```python
from build123d import *

# Parameters (mm, degrees)
SKETCH1_W           = 50
SKETCH1_H           = 21
BOSS_EXTRUDE1_DEPTH = 58
SKETCH3_R           = 7.5
CUT_EXTRUDE1_DEPTH  = 24
CUT_EXTRUDE2_REACH  = 66.025
SKETCH4_R           = 5.2
CUT_EXTRUDE3_START  = -24
SKETCH5_R           = 7.5
CUT_EXTRUDE3_DEPTH  = 24
CUT_EXTRUDE4_REACH  = 66.025
SKETCH6_R           = 4.5
CUT_EXTRUDE5_REACH  = 68.558
SKETCH8_W           = 10
SKETCH8_H           = 20
SKETCH11_W          = 4
SKETCH11_H          = 20
BOSS_EXTRUDE2_DEPTH = 26
SKETCH12_W          = 18
SKETCH12_H          = 20
BOSS_EXTRUDE3_DEPTH = 4
CUT_EXTRUDE7_DEPTH  = 79.487260113
FILLET1_R           = 5
SKETCH14_R          = 1.95
CUT_EXTRUDE8_DEPTH  = 10
SKETCH15_W          = 5.527864045
SKETCH15_H          = 1
CUT_EXTRUDE9_DEPTH  = 76.028327984
SKETCH17_W          = 30
SKETCH17_H          = 19
BOSS_EXTRUDE5_DEPTH = 18
SKETCH7_R           = 4.125
CUT_EXTRUDE6_DEPTH  = 45
FILLET8_R           = 3
SKETCH18_W          = 6
SKETCH18_H          = 5.5
CUT_EXTRUDE10_DEPTH = 1


with BuildPart() as part:
    # Sketch1 → Boss-Extrude1 (new body)
    with BuildSketch(Plane(origin=(0, 0, 0), x_dir=(1, 0, 0), z_dir=(0, 1, 0))):
        Rectangle(SKETCH1_W, SKETCH1_H)
    extrude(amount=BOSS_EXTRUDE1_DEPTH)

    # Sketch3 → Cut-Extrude1 (cut)
    with BuildSketch(Plane(origin=(0, 58, 0), x_dir=(1, 0, 0), z_dir=(0, 1, 0))):
        with Locations(Location((-15, 0, 0), (0, 0, 270))):
            Circle(SKETCH3_R)
    extrude(amount=-CUT_EXTRUDE1_DEPTH, mode=Mode.SUBTRACT)

    # Sketch4 → Cut-Extrude2 (cut, up to next)
    with BuildSketch(Plane(origin=(0, 58, 0), x_dir=(1, 0, 0), z_dir=(0, 1, 0)), mode=Mode.PRIVATE) as cut_extrude2_sk1:
        with Locations(Location((15, 0, 0), (0, 0, 270))):
            Circle(SKETCH4_R)
    cut_extrude2_tool1 = extrude(cut_extrude2_sk1.sketch, amount=-CUT_EXTRUDE2_REACH, mode=Mode.PRIVATE) & part.part
    add(cut_extrude2_tool1.solids().sort_by_distance((15, 58, 0))[0], mode=Mode.SUBTRACT)

    # Sketch5 → Cut-Extrude3 (cut)
    with BuildSketch(Plane.XZ.offset(CUT_EXTRUDE3_START)):
        with Locations(Location((-15, 0, 0), (0, 0, 90))):
            Circle(SKETCH5_R)
    extrude(amount=CUT_EXTRUDE3_DEPTH, mode=Mode.SUBTRACT)

    # Sketch6 → Cut-Extrude4 (cut, up to next)
    with BuildSketch(Plane.XZ, mode=Mode.PRIVATE) as cut_extrude4_sk1:
        with Locations(Location((-15, 0, 0), (0, 0, 270))):
            Circle(SKETCH6_R)
    cut_extrude4_tool1 = extrude(cut_extrude4_sk1.sketch, amount=-CUT_EXTRUDE4_REACH, mode=Mode.PRIVATE) & part.part
    add(cut_extrude4_tool1.solids().sort_by_distance((-15, 0, 0))[0], mode=Mode.SUBTRACT)

    # Sketch8 → Cut-Extrude5 (cut, up to next)
    with BuildSketch(Plane.XY.offset(10.5), mode=Mode.PRIVATE) as cut_extrude5_sk1:
        with Locations((0, 29)):
            Rectangle(SKETCH8_W, SKETCH8_H)
    cut_extrude5_tool1 = extrude(cut_extrude5_sk1.sketch, amount=-CUT_EXTRUDE5_REACH, mode=Mode.PRIVATE) & part.part
    add(cut_extrude5_tool1.solids().sort_by_distance((0, 29, 10.5))[0], mode=Mode.SUBTRACT)

    # Sketch11 → Boss-Extrude2 (add)
    with BuildSketch(Plane(origin=(0, 0, -10.5), x_dir=(-1, 0, 0), z_dir=(0, 0, -1))):
        with Locations((7, 29)):
            Rectangle(SKETCH11_W, SKETCH11_H)
        with Locations((-7, 29)):
            Rectangle(SKETCH11_W, SKETCH11_H)
    extrude(amount=BOSS_EXTRUDE2_DEPTH)

    # Sketch12 → Boss-Extrude3 (add)
    with BuildSketch(Plane(origin=(0, 0, -36.5), x_dir=(-1, 0, 0), z_dir=(0, 0, -1))):
        with Locations((0, 29)):
            Rectangle(SKETCH12_W, SKETCH12_H)
    extrude(amount=BOSS_EXTRUDE3_DEPTH)

    # Sketch13 → Cut-Extrude7 (cut, through all)
    with BuildSketch(Plane(origin=(9, 0, 0), x_dir=(0, 0, -1), z_dir=(1, 0, 0))):
        with BuildLine():
            Line((18.25, 31.75), (27.25, 31.75))
            ThreePointArc((27.25, 31.75), (30, 29), (27.25, 26.25))
            Line((27.25, 26.25), (18.25, 26.25))
            ThreePointArc((18.25, 26.25), (15.5, 29), (18.25, 31.75))
        make_face()
    extrude(amount=-CUT_EXTRUDE7_DEPTH, mode=Mode.SUBTRACT)

    # Fillet1
    fillet1_edges = [part.edges().sort_by_distance(p)[0] for p in [
        (25, 29, 10.5),
        (-25, 29, 10.5),
    ]]
    fillet(fillet1_edges, radius=FILLET1_R)

    # Sketch14 → Cut-Extrude8 (cut)
    with BuildSketch(Plane.XZ):
        with Locations(Location((20.550788232, 5.550788232, 0), (0, 0, 270))):
            Circle(SKETCH14_R)
        with Locations(Location((9.449211768, -5.550788232, 0), (0, 0, 270))):
            Circle(SKETCH14_R)
    extrude(amount=-CUT_EXTRUDE8_DEPTH, mode=Mode.SUBTRACT)

    # Sketch15 → Cut-Extrude9 (cut, through all)
    with BuildSketch(Plane(origin=(0, 58, 0), x_dir=(1, 0, 0), z_dir=(0, 1, 0))):
        with Locations((-22.236067977, 0)):
            Rectangle(SKETCH15_W, SKETCH15_H)
    extrude(amount=-CUT_EXTRUDE9_DEPTH, mode=Mode.SUBTRACT)

    # Sketch17 → Boss-Extrude5 (add)
    with BuildSketch(Plane(origin=(9, 0, 0), x_dir=(0, 0, -1), z_dir=(1, 0, 0))):
        with Locations((25.5, 48.5)):
            Rectangle(SKETCH17_W, SKETCH17_H)
        with Locations((25.5, 9.5)):
            Rectangle(SKETCH17_W, SKETCH17_H)
    extrude(amount=-BOSS_EXTRUDE5_DEPTH)

    # Sketch7 → Cut-Extrude6 (cut)
    with BuildSketch(Plane.XY.offset(10.5)):
        with Locations((0, 49)):
            Circle(SKETCH7_R)
        with Locations((0, 9)):
            Circle(SKETCH7_R)
    extrude(amount=-CUT_EXTRUDE6_DEPTH, mode=Mode.SUBTRACT)

    # Fillet8
    fillet8_edges = [part.edges().sort_by_distance(p)[0] for p in [
        (-9, 29, -40.5),
        (9, 29, -40.5),
    ]]
    fillet(fillet8_edges, radius=FILLET8_R)

    # Sketch18 → Cut-Extrude10 (cut)
    with BuildSketch(Plane(origin=(0, 0, -40.5), x_dir=(-1, 0, 0), z_dir=(0, 0, -1))):
        with Locations((0, 29)):
            Rectangle(SKETCH18_W, SKETCH18_H)
    extrude(amount=-CUT_EXTRUDE10_DEPTH, mode=Mode.SUBTRACT)


solid = part.part
```
The model under review builds one solid part; all positions refer to its coordinate system, in mm. A direction names the side the tool comes from. Round coordinates to 2 decimals unless told otherwise and drop trailing zeros. Order: outer loops, then holes, each group sorted by start corner. A loop starts at its lowest first (then second) coordinate and runs counter-clockwise, first axis right, second up. Notation, with made-up numbers: (-11.5, 38.25) - (43.5, 38.25) arc R22 ccw to (43.5, 76.25) - close; hole circle Ø5 at (-3, -32). An arc over 180 degrees is marked (long way). Answer in a Markdown table with one row per item.
(1) Take a section at D-D on x = -17.5. Write out the cut boundary in (y, z).
Result set:
| item | result |
|---|---|
| outline | (0, -10.5) - (58, -10.5) - (58, -7.07) - (34, -7.07) - (34, -3.74) - (24, -3.74) - (24, -7.07) - (0, -7.07) - close; (0, 7.07) - (24, 7.07) - (24, 3.74) - (34, 3.74) - (34, 7.07) - (58, 7.07) - (58, 10.5) - (0, 10.5) - close |
(2) Mouldability with a two-part tool opening along X and no side actions: class faces 1 (the face through (-23.57, 29.41, 9)), 2 (the face through (-17, 29, -10.5)), 3 (the face through (0, 29, -39.5)), 4 (the face through (-1, 45, -12)) as released by +X, released by -X, zero draft, split by the parting line, or undercut.
Result set:
| item | result |
|---|---|
| face 1 | released by -X |
| face 2 | zero draft |
| face 3 | undercut |
| face 4 | undercut |
(3) Take a section at C-C on x = 0. Write out the cut boundary in (y, z) (3 decimals), plus the area to 3 significant figures.
Result set:
| item | result |
|---|---|
| outline | (0, -40.5) - (26.25, -40.5) - (26.25, -39.5) - (31.75, -39.5) - (31.75, -40.5) - (58, -40.5) - (58, 10.5) - (53.125, 10.5) - (53.125, -34.5) - (44.875, -34.5) - (44.875, 10.5) - (39, 10.5) - (39, -36.5) - (19, -36.5) - (19, 10.5) - (13.125, 10.5) - (13.125, -34.5) - (4.875, -34.5) - (4.875, 10.5) - (0, 10.5) - close |
| area | 1,270 mm2 |
(4) Take a section at B-B on y = 49. Write out the cut boundary in (x, z) (3 decimals), plus the area to 3 significant figures.
Result set:
| item | result |
|---|---|
| outline | (-25, -10.5) - (-9, -10.5) - (-9, -37.5) arc R3 ccw to (-6, -40.5) - (6, -40.5) arc R3 ccw to (9, -37.5) - (9, -10.5) - (25, -10.5) - (25, 5.5) arc R5 ccw to (20, 10.5) - (4.125, 10.5) - (4.125, -34.5) - (-4.125, -34.5) - (-4.125, 10.5) - (-20, 10.5) arc R5 ccw to (-25, 5.5) - (-25, 0.5) - (-22.483, 0.5) arc R7.5 cw (long way) to (-22.483, -0.5) - (-25, -0.5) - close; hole circle Ø10.4 at (15, 0) |
| area | 940 mm2 |
(5) Take a section at A-A on z = -12.5. Write out the cut boundary in (x, y) (3 decimals).
Result set:
| item | result |
|---|---|
| outline | (-9, 0) - (9, 0) - (9, 58) - (-9, 58) - close; hole (-5, 19) - (5, 19) - (5, 39) - (-5, 39) - close; hole circle Ø8.25 at (0, 9); hole circle Ø8.25 at (0, 49) |
(6) Clearance check with flat-ended pins moving along their axes: P1, Ø17.5, axis at x = -17.5, y = 39.5, coming from the -Z side; P2, Ø3, axis at x = 11, y = 9.5, coming from the -Z side; P3, Ø2.5, axis at x = 20.55, z = 5.55, coming from the -Y side. State where each tip first meets the part, or that it passes through.
Result set:
| item | result |
|---|---|
| P1 | stops at z = -38.7 |
| P2 | stops at z = -10.5 |
| P3 | stops at y = 10 |
(7) Machinability: for faces 5 (the face through (-7, 29, -30)), 6 (the face through (-24, 29, 0.5)), 7 (the face through (-1, 5, -12)), which of the approach directions +Z, -Z, +X, -X, +Y, -Y give a long, thin tool a straight path to every point of the face, cutting with its end or side? Answer none if there is none.
Result set:
| item | result |
|---|---|
| face 5 | +X, -X |
| face 6 | -X, +Y, -Y |
| face 7 | +Z |
(8) For line 1 (Y direction, x = 0, z = -14) (3 decimals); line 2 (Z direction, x = -15, y = 29); line 3 (Y direction, x = 2, z = -26), list the stretches that pass through material, from the lowest coordinate up. Write a range as from..to.
Result set:
| item | result |
|---|---|
| line 1 | y = 0..4.875, 13.125..19, 39..44.875, 53.125..58 |
| line 2 | z = -10.5..-4.5, 4.5..10.5 |
| line 3 | y = 0..5.39, 12.61..19, 39..45.39, 52.61..58 |
